The listing builds one solid part. Answer for the finished solid, in the listing's coordinates (mm). A direction names the side the tool comes from. Coordinates: 2 decimals unless noted, no trailing zeros. Order: outer loops, then holes, each group sorted by start corner. A loop starts at its lowest first (then second) coordinate and runs counter-clockwise, first axis right, second up. Notation, with made-up numbers: (22, -31) -> (55, -31) arc R29 ccw to (55, 6) -> close; hole circle Ø2 at (58.25, 13). An arc over 180 degrees is marked (long way). Return JSON: item names as keys, results as strings.
```python
from build123d import *

# Parameters (mm, degrees)
F1_DEPTH = 12.7


with BuildPart() as f1:
    # F0 (on Right) → F1 (new body)
    with BuildSketch(Plane.YZ):
        Polygon((-81.148056, 152.4), (-81.148056, 0), (-64.264163, 45.804784), (-57.39085, 6.09312), (-37.22056, -31.817149), (-37.22056, 35.310104), (-30.08927, 6.09312), (-19.019617, 33.24692), (-19.019617, -41.578095), (-8.49505, -19.859882), (4.483057, -102.9488), (9.243387, 6.09312), (21.866368, -155.964419), (28.112774, -139.018371), (28.112774, -174.600467), (33.099876, -161.07082), (37.128638, -223.373905), (46.750363, -174.600467), (53.567908, -218.248002), (61.619878, -180.88825), (69.072234, -228.6), (71.251944, -228.6), (71.251944, 152.4), align=None)
    extrude(amount=F1_DEPTH)


solid = f1.part
```
Item 1: The part is cut by section D-D on y = -15.5. Determine the outline of the cut face in (x, z).
Answer list:
{"outline": "(0, -34.32) -> (12.7, -34.32) -> (12.7, 152.4) -> (0, 152.4) -> close"}
Item 2: The part is cut by section A-A on x = 9.5. Determine the outline of the cut face in (y, z).
Answer list:
{"outline": "(-81.15, 0) -> (-64.26, 45.8) -> (-57.39, 6.09) -> (-37.22, -31.82) -> (-37.22, 35.31) -> (-30.09, 6.09) -> (-19.02, 33.25) -> (-19.02, -41.58) -> (-8.5, -19.86) -> (4.48, -102.95) -> (9.24, 6.09) -> (21.87, -155.96) -> (28.11, -139.02) -> (28.11, -174.6) -> (33.1, -161.07) -> (37.13, -223.37) -> (46.75, -174.6) -> (53.57, -218.25) -> (61.62, -180.89) -> (69.07, -228.6) -> (71.25, -228.6) -> (71.25, 152.4) -> (-81.15, 152.4) -> close"}
Item 3: Determine the mould class of faces 3 (the flat face through (6.261, 57.538, -199.83)), 4 (the flat face through (6, 71.252, -41)), 5 (the flat face through (6, -4, 152.4)) for opening direction Y: pulls with the +Y half, pulls with the -Y half, needs draft (parallel to the pull), parting line crosses it, or undercut.
Answer list:
{"face 3": "undercut", "face 4": "pulls with the +Y half", "face 5": "needs draft"}
Item 4: Find the intervals of material crossed by probe 1 along Y at (x, z) = (5.75, -30); probe 2 along Y at (x, z) = (10, -192); probe 3 along Y at (x, z) = (6, -184), in increasing order.
Answer list:
{"probe 1": "-38.19 to -37.22, -19.02 to -13.41, -6.91 to 7.67, 12.05 to 71.25", "probe 2": "35.1 to 43.32, 49.47 to 59.23, 63.36 to 71.25", "probe 3": "34.58 to 44.9, 48.22 to 60.95, 62.11 to 71.25"}
Item 5: The part is cut by section B-B on z = -25.5. Determine the outline of the cut face in (x, y), plus the area to 3 significant figures.
Answer list:
{"outline": "(0, -40.58) -> (12.7, -40.58) -> (12.7, -37.22) -> (0, -37.22) -> close; (0, -19.02) -> (12.7, -19.02) -> (12.7, -11.23) -> (0, -11.23) -> close; (0, -7.61) -> (12.7, -7.61) -> (12.7, 7.86) -> (0, 7.86) -> close; (0, 11.7) -> (12.7, 11.7) -> (12.7, 71.25) -> (0, 71.25) -> close", "area": "1,090 mm2"}
Item 6: Which of the six approach directions +Z, -Z, +X, -X, +Y, -Y give full straight-line access (tool end or side, diameter ignored) to faces 1 (the flat face through (0, 11, 49)), 2 (the flat face through (6, -19.02, -4))?
Answer list:
{"face 1": "+Z, -Z, -X, +Y, -Y", "face 2": "-Z, +X, -X"}
Item 7: Flat-ended cylindrical pins translate along their axes: pin 1 (2 mm diameter, centred on x = 8, y = -39.5, fed in from -Z); pin 2 (1 mm diameter, centred on x = 4, z = -170, fed in from -Y). Find the tip coordinate at first contact, or state that the pin passes through.
Answer list:
{"pin 1": "z = -29.41", "pin 2": "y = 28.11"}
Item 8: The part is cut by section C-C on z = -202. Determine the outline of the cut face in (x, y).
Answer list:
{"outline": "(0, 35.75) -> (12.7, 35.75) -> (12.7, 41.35) -> (0, 41.35) -> close; (0, 51.03) -> (12.7, 51.03) -> (12.7, 57.07) -> (0, 57.07) -> close; (0, 64.92) -> (12.7, 64.92) -> (12.7, 71.25) -> (0, 71.25) -> close"}
